```python
from build123d import *

# Parameters (mm, degrees)
F0_W        = 11.2655872395
F0_H        = 11.2655872395
F0_R        = 2.15265
F1_DEPTH    = 22.4125
F2_W        = 11.2655872395
F2_H        = 11.2655872395
F3_DEPTH    = 1.5875
F4_W        = 11.2655872395
F4_H        = 11.2655872395
F4_R        = 2.15265
F5_DEPTH    = 12.7
F6_R        = 1.35255
F7_DEPTH    = 4.9581264334
F8_T1_DEPTH = 64.8639645


# Not quite as in the source:
# - a fillet or chamfer that OpenCascade refuses, or shapes differently, is made with other operations: its cross-section is extruded or revolved along the edge and cut away or added


with BuildPart() as f1:
    # F0 (on Top) → F1 (new body)
    with BuildSketch(Plane.XY):
        Rectangle(F0_W, F0_H)
        Circle(F0_R, mode=Mode.SUBTRACT)
    extrude(amount=F1_DEPTH)

    # F2 (on face) → F3 (join)
    with BuildSketch(Plane.XY.offset(22.4125)):
        Rectangle(F2_W, F2_H)
    extrude(amount=F3_DEPTH)

    # F4 (on face) → F5 (join)
    with BuildSketch(Plane.XY.offset(24)):
        Rectangle(F4_W, F4_H)
        Circle(F4_R, mode=Mode.SUBTRACT)
    extrude(amount=F5_DEPTH)

    # F6 (on face) → F7 (cut, up to face)
    with BuildSketch(Plane(origin=(-5.6327936197, 0, 0), x_dir=(0, -1, 0), z_dir=(-1, 0, 0))):
        with Locations((0, 11.20625)):
            Circle(F6_R)
        with Locations((0, 30.35)):
            Circle(F6_R)
    extrude(amount=-F7_DEPTH, mode=Mode.SUBTRACT)

    # F8: fillet of radius 5.6327929 on 4 edges, made by hand

    # F8_s2 → F8_t1 (cut)
    with BuildSketch(Plane.XY.offset(-14.08198225)):
        with BuildLine():
            ThreePointArc((-5.6327936197, 7.197e-07), (-3.9829867763, 3.9829867763), (-7.197e-07, 5.6327936197))
            Line((-7.197e-07, 5.6327936197), (-5.6327936197, 5.6327936197))
            Line((-5.6327936197, 5.6327936197), (-5.6327936197, 7.197e-07))
        make_face()
        with BuildLine():
            ThreePointArc((5.6327936197, 7.197e-07), (3.9829867763, 3.9829867763), (7.197e-07, 5.6327936197))
            Line((7.197e-07, 5.6327936197), (5.6327936197, 5.6327936197))
            Line((5.6327936197, 5.6327936197), (5.6327936197, 7.197e-07))
        make_face()
        with BuildLine():
            ThreePointArc((-7.197e-07, -5.6327936197), (-3.9829867763, -3.9829867763), (-5.6327936197, -7.197e-07))
            Line((-5.6327936197, -7.197e-07), (-5.6327936197, -5.6327936197))
            Line((-5.6327936197, -5.6327936197), (-7.197e-07, -5.6327936197))
        make_face()
        with BuildLine():
            ThreePointArc((7.197e-07, -5.6327936197), (3.9829867763, -3.9829867763), (5.6327936197, -7.197e-07))
            Line((5.6327936197, -7.197e-07), (5.6327936197, -5.6327936197))
            Line((5.6327936197, -5.6327936197), (7.197e-07, -5.6327936197))
        make_face()
    extrude(amount=F8_T1_DEPTH, mode=Mode.SUBTRACT)


solid = f1.part
```
Here's how the part is built. I have some questions about the finished solid (model axes, mm). A direction names the side the tool comes from. Coordinates: 2 decimals unless noted, no trailing zeros. Order: outer loops, then holes, each group sorted by start corner. A loop starts at its lowest first (then second) coordinate and runs counter-clockwise, first axis right, second up.
Item 1: I need wall thicknesses on probe 1 along Z at (x, y) = (-4.5, -0.75); probe 2 along Z at (x, y) = (-5, -1); probe 3 along Z at (x, y) = (-1.25, -1.5). Which ranges of each line are inside material? Lowest first, please.
Response values:
probe 1: z = 0 to 10.08, 12.33 to 29.22, 31.48 to 36.7
probe 2: z = 0 to 10.3, 12.12 to 29.44, 31.26 to 36.7
probe 3: z = 22.41 to 24
Item 2: If we section it at C-C, the plane x = -2.75: List the corners of the cut face in (y, z) for me.
Response values:
outline: (-4.92, 0) - (4.92, 0) - (4.92, 36.7) - (-4.92, 36.7) - close; hole circle Ø2.71 at (0, 11.21); hole circle Ø2.71 at (0, 30.35)
Item 3: If we section it at B-B, the plane y = -0.75: List the corners of the cut face in (x, z) for me, then the cut area to 3 significant figures.
Response values:
outline: (-5.58, 0) - (-2.02, 0) - (-2.02, 10.08) - (-5.58, 10.08) - close; (-5.58, 12.33) - (-2.02, 12.33) - (-2.02, 22.41) - (2.02, 22.41) - (2.02, 0) - (5.58, 0) - (5.58, 36.7) - (2.02, 36.7) - (2.02, 24) - (-2.02, 24) - (-2.02, 29.22) - (-5.58, 29.22) - close; (-5.58, 31.48) - (-2.02, 31.48) - (-2.02, 36.7) - (-5.58, 36.7) - close
area: 252 mm2
Item 4: I'm going to push flat-ended pins straight in: pin 1 Ø5 at (x, z) = (-2, 10) entering from -Y; pin 2 Ø2 at (y, z) = (-1.5, 24) entering from -X; pin 3 Ø2 at (x, y) = (0, 1) entering from -Z; pin 4 Ø2 at (x, y) = (0.5, -1) entering from +Z. Where does each tip first touch, or does it pass through?
Response values:
pin 1: stops at y = -5.63
pin 2: stops at x = -5.61
pin 3: stops at z = 22.41
pin 4: stops at z = 24
Item 5: Thinking about a two-plate mould opening in X: for faces 1 (the face through (-4.027, 3.939, 18.093)), 2 (the face through (-0.1, -2.4, 0)), 3 (the face through (0, 0, 24)), which applies, pulls with the +X half, pulls with the -X half, needs draft (parallel to the pull), parting line crosses it, or undercut?
Response values:
face 1: pulls with the -X half
face 2: needs draft
face 3: undercut
Item 6: Which directions (+Z, -Z, +X, -X, +Y, -Y) give clear straight access to the entire face, cutting with the end or side of a thin tool? Please do faces 4 (the face through (-3.68, 1.35, 11.27)), 5 (the face through (2.053, 0.647, 30.261)), 6 (the face through (0, 0, 22.412)).
Response values:
face 4: -X
face 5: +Z
face 6: -Z
